Can you work these out from the model? Positions are in its coordinate system, mm. Face numbers are marked on the shaded views. A direction names the side the tool comes from. Give positions to 0.01 mm unless a question says otherwise; leave off trailing zeros. Write each loop counter-clockwise with the first axis right and the second up, starting at its lowest first coordinate (ties: lowest second). Pieces come first, ordered by that corner, then holes.
1. On a 3-axis mill with a long thin cutter (end or side, diameter ignored), from which of +Z, -Z, +X, -X, +Y, -Y can I reach the whole of each face in a straight line? I mean the marked faces 1, 2 and 3. Say none if no direction works.
2. I'm going to push flat-ended pins straight in: pin 1 (2.5 mm diameter, centred on x = -23, y = -1, fed in from -Z); pin 2 (6 mm diameter, centred on x = 5, y = -1, fed in from +Z); pin 3 (3 mm diameter, centred on x = 25, y = 0, fed in from -Z); pin 4 (2 mm diameter, centred on y = -4, z = 1, fed in from -X). Where does each tip first touch, or does it pass through?
3. Suppose I cut it at B-B (x = -10.5). Please give me the cut outline in (y, z), and give its area (3 significant figures).
4. Thinking about a two-plate mould opening in X: for the marked faces 4 and 5, which applies, pulls with the +X half, pulls with the -X half, needs draft (parallel to the pull), parting line crosses it, or undercut?
5. If I drill on probe 1 along X at (y, z) = (0, 2); probe 2 along X at (y, z) = (0, 5.85); probe 3 along Y at (x, z) = (25, 5.35), over which ranges is the centre line in solid material (lowest first)?
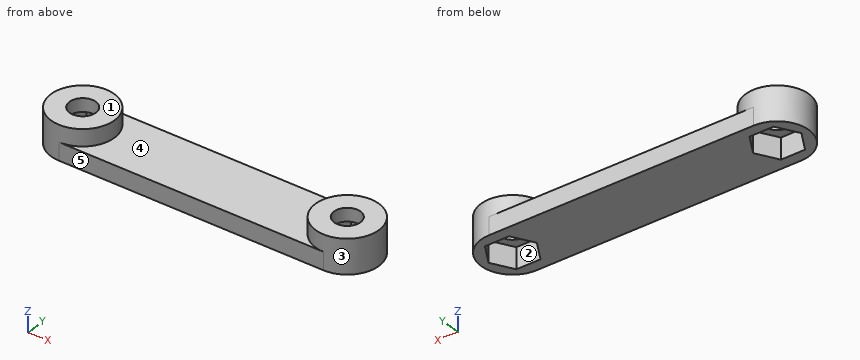
```python
from build123d import *

# Parameters (mm, degrees)
SKETCH1_R           = 2.5
BOSS_EXTRUDE1_DEPTH = 3.35
SKETCH2_R           = 6
SKETCH2_R_2         = 2.5
BOSS_EXTRUDE2_DEPTH = 3.15
CUT_EXTRUDE1_DEPTH  = 4


with BuildPart() as part:
    # Sketch1 → Boss-Extrude1 (new body)
    with BuildSketch(Plane.XY):
        with BuildLine():
            Line((-25, -6), (25, -6))
            ThreePointArc((25, -6), (31, 0), (25, 6))
            Line((25, 6), (-25, 6))
            ThreePointArc((-25, 6), (-31, 0), (-25, -6))
        make_face()
        with Locations((-25, 0)):
            Circle(SKETCH1_R, mode=Mode.SUBTRACT)
        with Locations((25, 0)):
            Circle(SKETCH1_R, mode=Mode.SUBTRACT)
    extrude(amount=BOSS_EXTRUDE1_DEPTH)

    # Sketch2 → Boss-Extrude2 (add)
    # profile 1 of 2: a face of its own
    with BuildSketch(Plane.XY.offset(3.35)):
        with Locations(Location((-25, 0, 0), (0, 0, 270))):
            Circle(SKETCH2_R)
        with Locations((-25, 0)):
            Circle(SKETCH2_R_2, mode=Mode.SUBTRACT)
    # profile 2 of 2: a face of its own
    with BuildSketch(Plane.XY.offset(3.35)):
        with Locations(Location((25, 0, 0), (0, 0, 90))):
            Circle(SKETCH2_R)
        with Locations((25, 0)):
            Circle(SKETCH2_R_2, mode=Mode.SUBTRACT)
    extrude(amount=BOSS_EXTRUDE2_DEPTH)

    # Sketch3 → Cut-Extrude1 (cut)
    with BuildSketch(Plane(origin=(0, 0, 0), x_dir=(-1, 0, 0), z_dir=(0, 0, -1))):
        Polygon((20.438932873, 0), (22.719466437, 3.95), (27.280533563, 3.95), (29.561067127, 0), (27.280533563, -3.95), (22.719466437, -3.95), align=None)
        Polygon((-22.719466437, 3.95), (-27.280533563, 3.95), (-29.561067127, 0), (-27.280533563, -3.95), (-22.719466437, -3.95), (-20.438932873, 0), align=None)
    extrude(amount=-CUT_EXTRUDE1_DEPTH, mode=Mode.SUBTRACT)


solid = part.part
```
Checks:
1. face 1: +Z, +X, -X, +Y, -Y
1. face 2: -Z
1. face 3: +Z
2. pin 1: stops at z = 4
2. pin 2: stops at z = 3.35
2. pin 3: passes through
2. pin 4: stops at x = -30.2
3. outline: (-6, 0) - (6, 0) - (6, 3.35) - (-6, 3.35) - close
3. area: 40.2 mm2
4. face 4: undercut
4. face 5: needs draft
5. probe 1: x = -31 to -29.56, -20.44 to 20.44, 29.56 to 31
5. probe 2: x = -31 to -27.5, -22.5 to -19, 19 to 22.5, 27.5 to 31
5. probe 3: y = -6 to -2.5, 2.5 to 6
